Autodesk Inventor part; units mm, degrees
ref_plane "YZ Plane" through (0, 0, 0) normal (1, 0, 0) x (0, 1, 0)
ref_plane "XZ Plane" through (0, 0, 0) normal (0, 1, 0) x (-1, 0, 0)
ref_plane "XY Plane" through (0, 0, 0) normal (0, 0, 1) x (1, 0, 0)
sketch "Sketch1" plane through (0, 0, 0) normal (0, 0, 1) x (1, 0, 0)
  line L0 (-5.334, 0) -> (5.334, 0)
  line L1 (0, -4.572) -> (0, 27.432)
  line L2 (3.81, 0) -> (-3.81, 0)
  line L3 (-3.81, 0) -> (-3.81, 20.6603)
  line L4 (3.81, 20.6603) -> (3.81, 0)
  line L5 (-3.81, 20.6603) -> (-2.54, 22.86)
  line L6 (-2.54, 22.86) -> (2.54, 22.86)
  line L7 (2.54, 22.86) -> (3.81, 20.6603)
  point P0 (0, 0)
  point P1 (0, 0)
  point P2 (0, 22.86)
  dimension "d0" = 22.86
  dimension "d1" = 5.08
  dimension "d2" = 60
  dimension "d3" = 7.62
extrude "Extrusion1" add sketch "Sketch1" against normal blind 2.54
sketch "Sketch2" plane through (0, 0, 0) normal (0, 0, 1) x (1, 0, 0)
  line L0 (0, -4.572) -> (0, 27.432)
  line L1 (2.54, 22.86) -> (-2.54, 22.86)
  point P0 (0, 0)
  point P1 (0, 14.7066)
  dimension "d18" = 8.1534
hole "Hole1" at (0, 14.7066, 0) direction (0, 0, -1) diameter 3.175 end through all
fillet "Fillet1" radius 3.175 4 edges at (3.81, 0, -1.27) (-3.81, 0, -1.27) (3.81, 20.6603, -1.27) (-3.81, 20.6603, -1.27)
sketch "Sketch3" plane through (0, 0, 0) normal (0, 0, 1) x (1, 0, 0)
  point P0 (0, 0)
  point P1 (0, 3.302)
  dimension "d31" = 3.302
hole "Hole3" at (0, 3.302, 0) direction (0, 0, -1) diameter 1.7018 end through all
properties part number "plate_02 for metal"
CAD build for the part. Positions are in the model's coordinates, mm. Coordinates: 2 decimals unless noted, no trailing zeros. Order: outer loops, then holes, each group sorted by start corner. A loop starts at its lowest first (then second) coordinate and runs counter-clockwise, first axis right, second up.
Item 1: Band-saw the part on D-D on x = 3. List the corners of the cut face in (y, z).
Check sheet entries:
outline: (1.06, -2.54) - (22.06, -2.54) - (22.06, 0) - (1.06, 0) - close
Item 2: Band-saw the part on B-B on z = -0.95. Give the number of separate pieces and of enclosed holes in the cut face, plus the area to 3 significant figures.
Check sheet entries:
separate pieces: 1
enclosed holes: 2
area: 157 mm2
Item 3: Two-plate mould, pull along X, no slides. Class faces 1 (the face through (2.9, 0.95, -1.29)), 2 (the face through (0.61, 13.24, -1.29)), 3 (the face through (-2.86, 0.91, -1.29)): +X half, -X half, draft (parallel to the pull), parting line (faces both ways), or undercut.
Check sheet entries:
face 1: +X half
face 2: undercut
face 3: -X half
Item 4: Band-saw the part on A-A on x = 0. List the corners of the cut face in (y, z), plus the area to 3 significant figures.
Check sheet entries:
outline: (0, -2.54) - (2.45, -2.54) - (2.45, 0) - (0, 0) - close; (4.15, -2.54) - (13.12, -2.54) - (13.12, 0) - (4.15, 0) - close; (16.29, -2.54) - (22.86, -2.54) - (22.86, 0) - (16.29, 0) - close
area: 45.7 mm2
Item 5: Band-saw the part on C-C on x = -1.25. List the corners of the cut face in (y, z), plus the area to 3 significant figures.
Check sheet entries:
outline: (0.06, -2.54) - (13.73, -2.54) - (13.73, 0) - (0.06, 0) - close; (15.69, -2.54) - (22.86, -2.54) - (22.86, 0) - (15.69, 0) - close
area: 52.9 mm2
Item 6: Pin check, flat tip, straight feed: pin 1 Ø2 at (x, y) = (0, 14.5) entering from -Z. Stop position of the tip, or through.
Check sheet entries:
pin 1: passes through
Item 7: Drill centre lines: L1, parallel to Y at x = 0, z = -1.2; L2, parallel to X at y = 13.25, z = -1.65; L3, parallel to X at y = 3.25, z = -1.4. Where is each one in solid material? Low to high.
Check sheet entries:
L1: y = 0 to 2.45, 4.15 to 13.12, 16.29 to 22.86
L2: x = -3.81 to -0.63, 0.63 to 3.81
L3: x = -3.81 to -0.85, 0.85 to 3.81
